Autodesk Inventor part; units mm, degrees
ref_plane "Work Plane2" through (0, 0, -28.5) normal (0.5, -0.866, 0) x (0, 0, 1)
ref_plane "Work Plane3" through (0, 0, -28.5) normal (1, 0, 0) x (0, 0, 1)
ref_plane "YZ Plane" through (0, 0, 0) normal (1, 0, 0) x (0, 1, 0)
sketch "Sketch1" plane through (0, 0, 0) normal (0, 1, 0) x (-1, 0, 0)
  line L0 (0, 0) -> (0, -30)
  line L1 (0, 0) -> (30, 0) construction
  spline S0 degree 2 poles (0, -30) (-5.2172, -27.9207) (-10.8719, -12.7372) knots 0 0 0 1 1 1
  line L2 (-10.8719, -12.7372) -> (-12.8062, 1.9407) construction
  line L3 (-12.8062, 1.9407) -> (0, 0) construction
  spline S1 degree 2 poles (-10.8719, -12.7372) (-12.8062, 1.9407) (0, 0) knots 1 1 1 2 2 2
  point P0 (-3.8105, -26.8078)
  dimension "d16" = 30
  dimension "d17" = 90
revolve "Revolution3" add sketch "Sketch1" angle 60 about axis through (0, 0, 0) along (0, 0, 1)
sketch "Sketch6" plane through (0, 0, -30) normal (0, -1, 0) x (1, 0, 0)
  line L0 (0, 30) -> (0, 27)
  line L1 (0, 30) -> (0, 0)
  line L2 (0, 27) -> (15, 27)
  line L3 (0, 0) -> (0, 1.5)
  spline S0 degree 3 poles (0, 1.5) (5.1775, 3.9151) (12.4804, 18.8279) (7.9089, 27) knots 0 0 0 0 1 1 1 1
  point P0 (4.4382, 5.8918)
  point P1 (8.9326, 16.7012)
  dimension "d19" = 3
  dimension "d20" = 15
  dimension "d21" = 1.5
revolve "Revolution4" cut sketch "Sketch6" angle 360 about axis through (0, 0, 0) along (0, 0, -1)
sketch "Sketch7" plane through (0, 0, -3) normal (0, -1, 0) x (1, 0, 0)
  line L0 (0, 3) -> (0, 0)
  line L1 (0, 0) -> (13, 0)
  line L2 (13, 0) -> (13, 5)
  line L3 (13, 5) -> (0, 5)
  line L4 (0, 5) -> (0, 0)
  dimension "d23" = 13
  dimension "d24" = 5
revolve "Revolution5" cut sketch "Sketch7" angle 360 about axis through (0, 0, 0) along (0, 0, -1)
sketch "Sketch8" plane through (0, 0, -30) normal (-0.866, 0.5, 0) x (0, 0, 1)
  line L0 (1.5, 0) -> (0, 0)
  line L1 (1.5, 0) -> (30, 0)
ref_plane "Work Plane2" through (0, 0, -28.5) normal (0.5, -0.866, 0) x (0, 0, 1)
sketch "Sketch9" plane through (0, 0, -28.5) normal (0.5, -0.866, 0) x (0, 0, 1)
  line L0 (25.5, -6.8493) -> (25.5, -8.3976)
  line L1 (25.5, -7.9089) -> (25.5, -6.8493)
  line L2 (25.5, -8.3976) -> (25.5, -7.9089)
  line L3 (25.5, -7.9089) -> (25.5, -13.2779)
  line L4 (25.5, -7.9089) -> (29.8301, -5.4089)
  line L5 (25.5, -7.9089) -> (30.5, -7.9089) construction
  circle A0 centre (29.8301, -5.4089) radius 1.75
  circle A1 centre (29.8301, -5.4089) radius 1.05
  spline S0 degree 2 poles (30.7051, -6.9244) (27.615, -9.9944) (21.9704, -10.8927) knots 0 0 0 1 1 1
  spline S1 degree 3 poles (28.9551, -3.8934) (23.9976, -6.7492) (23.8027, -11.1988) (20.2008, -10.2065) knots 0 0 0 0 1 1 1 1
  line L6 (21.9704, -10.8927) -> (20.2008, -10.2065)
  point P0 (28.5, 0)
  point P1 (27.284, -9.3075)
  point P2 (24.5466, -7.9089)
  point P3 (22.5368, -9.9569)
  dimension "d27" = 5
  dimension "d28" = 30
  dimension "d29" = 3.5
  dimension "d30" = 2.1
extrude "Extrusion2" add sketch "Sketch9" along normal mid plane 3
ref_plane "Work Plane3" through (0, 0, -28.5) normal (1, 0, 0) x (0, 0, 1)
properties part number "Innter_petal"
The listing builds one solid part. Answer for the finished solid, in the listing's coordinates (mm). A direction names the side the tool comes from. Give positions to 0.01 mm unless a question says otherwise; leave off trailing zeros. Use one line per item in the form item = value. Start each with the question number.
(1) Flat-ended cylindrical pins translate along their axes: pin 1 Ø2 at (x, y) = (5.5, 8) entering from +Z; pin 2 Ø1 at (x, z) = (2, -4) entering from +Y; pin 3 Ø3 at (x, z) = (3, -21) entering from +Y. Find the tip coordinate at first contact, or state that the pin passes through.
(2) For faces 1 (the cylindrical face through (3.89, 2.27, 2.83)), 2 (the flat face through (9, 2, -3)), 3 (the flat face through (6, 7, -3)), determine the directions among +Z, -Z, +X, -X, +Y, -Y from which every point of the face is accessible in a straight line to the end or side of a thin tool.
(3) The mould has two halves that part along X. Classify faces 4 (the flat face through (4.47, 7.74, -15.44)), 5 (the cylindrical face through (4.95, 2.88, 2.33)), 6 (the flat face through (9, 0, -15)): released by +X, released by -X, zero draft, split by the parting line, or undercut.
(4) Consider line 1 (Z direction, x = 5, y = 2.5); line 2 (Z direction, x = 1.5, y = 1.25); line 3 (X direction, y = 4, z = -16.5). Determine where each line is inside the solid, lowest interval first. Write a range as from..to.
Ans:
q1.pin_1 = -3
q1.pin_2 = through
q1.pin_3 = 6.85
q2.face_1 = none
q2.face_2 = +Z, +X, -Y
q2.face_3 = +Z, -X, +Y
q3.face_4 = released by -X
q3.face_5 = undercut
q3.face_6 = zero draft
q4.line_1 = -24.22..-22.24, -1.84..0.29, 2.37..3.07
q4.line_2 = -28.78..-27.1
q4.line_3 = 7.05..8.5
